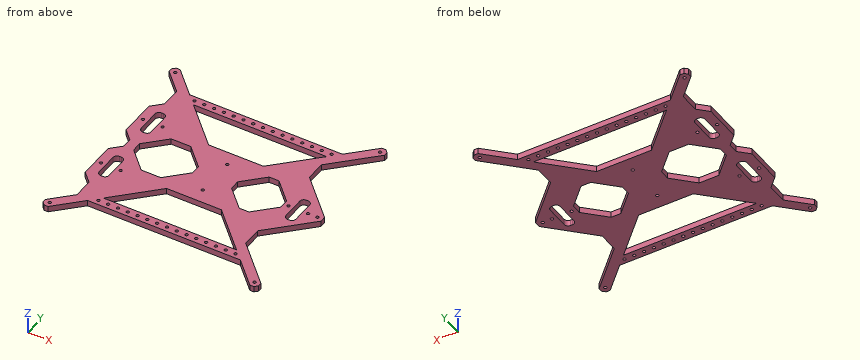
from build123d import *

# Parameters (mm, degrees)
MODEL_R                 = 1.5
SALIENTE_EXTRUIR1_DEPTH = 6
CROQUIS2_R              = 1.5
CROQUIS2_R_2            = 0.241728607
CORTAR_EXTRUIR1_DEPTH   = 7


with BuildPart() as part:
    # Model → Saliente-Extruir1 (new body)
    with BuildSketch(Plane.XY):
        Polygon((-105, 110), (-107, 110), (-110, 107), (-110, 105), (-110, 103), (-90, 83), (-90, 63), (-100, 53), (-100, 15), (-90, 5), (-90, -5), (-100, -15), (-100, -53), (-90, -63), (-90, -83), (-110, -103), (-110, -107), (-107, -110), (-105, -110), (-103, -110), (-78, -85), (78, -85), (103, -110), (105, -110), (107, -110), (110, -107), (110, -103), (90, -83), (70, -63), (70, -43), (90, -23), (110, -3), (110, 3), (90, 23), (70, 43), (70, 63), (110, 103), (110, 106), (110, 107), (107, 110), (103, 110), (80, 87), (78, 85), (-78, 85), (-103, 110), align=None)
        with Locations((104.5, 0)):
            Circle(MODEL_R, mode=Mode.SUBTRACT)
        with Locations((-95, 35)):
            Circle(MODEL_R, mode=Mode.SUBTRACT)
        with Locations((-75, 35)):
            Circle(MODEL_R, mode=Mode.SUBTRACT)
        with Locations((-95, -35)):
            Circle(MODEL_R, mode=Mode.SUBTRACT)
        with Locations((-75, -35)):
            Circle(MODEL_R, mode=Mode.SUBTRACT)
        with Locations((95, 0)):
            Circle(MODEL_R, mode=Mode.SUBTRACT)
        with Locations((75, 0)):
            Circle(MODEL_R, mode=Mode.SUBTRACT)
        with Locations((-104.5, 104.5)):
            Circle(MODEL_R, mode=Mode.SUBTRACT)
        with Locations((104.5, -104.5)):
            Circle(MODEL_R, mode=Mode.SUBTRACT)
        with Locations((104.5, 104.5)):
            Circle(MODEL_R, mode=Mode.SUBTRACT)
        with Locations((-104.5, -104.5)):
            Circle(MODEL_R, mode=Mode.SUBTRACT)
        with Locations((0, -20.5)):
            Circle(MODEL_R, mode=Mode.SUBTRACT)
        with Locations((0, 20.5)):
            Circle(MODEL_R, mode=Mode.SUBTRACT)
        Polygon((40, 47), (38, 45), (28, 35), (-28, 35), (-68, 75), (68, 75), align=None, mode=Mode.SUBTRACT)
        Polygon((28, -35), (-28, -35), (-68, -75), (68, -75), align=None, mode=Mode.SUBTRACT)
        Polygon((-80, 5), (-60, 25), (-40, 25), (-20, 5), (-20, -5), (-40, -25), (-60, -25), (-80, -5), align=None, mode=Mode.SUBTRACT)
        Polygon((50, 25), (70, 5), (70, -5), (50, -25), (40, -25), (20, -5), (20, 5), (40, 25), align=None, mode=Mode.SUBTRACT)
        with BuildLine():
            Line((-90, -46), (-90, -23))
            ThreePointArc((-90, -23), (-88.828427125, -20.171572875), (-86, -19))
            Line((-86, -19), (-84, -19))
            ThreePointArc((-84, -19), (-81.171572875, -20.171572875), (-80, -23))
            Line((-80, -23), (-80, -46))
            ThreePointArc((-80, -46), (-81.171572875, -48.828427125), (-84, -50))
            Line((-84, -50), (-86, -50))
            ThreePointArc((-86, -50), (-88.828427125, -48.828427125), (-90, -46))
        make_face(mode=Mode.SUBTRACT)
        with BuildLine():
            Line((-90, 24.007036896), (-90, 47.007036896))
            ThreePointArc((-90, 47.007036896), (-88.828427125, 49.835464021), (-86, 51.007036896))
            Line((-86, 51.007036896), (-84, 51.007036896))
            ThreePointArc((-84, 51.007036896), (-81.171572875, 49.835464021), (-80, 47.007036896))
            Line((-80, 47.007036896), (-80, 24.007036896))
            ThreePointArc((-80, 24.007036896), (-81.171572875, 21.178609771), (-84, 20.007036896))
            Line((-84, 20.007036896), (-86, 20.007036896))
            ThreePointArc((-86, 20.007036896), (-88.828427125, 21.178609771), (-90, 24.007036896))
        make_face(mode=Mode.SUBTRACT)
        with BuildLine():
            Line((80, -12.137123607), (80, 10.862876393))
            ThreePointArc((80, 10.862876393), (81.171572875, 13.691303518), (84, 14.862876393))
            Line((84, 14.862876393), (86, 14.862876393))
            ThreePointArc((86, 14.862876393), (88.828427125, 13.691303518), (90, 10.862876393))
            Line((90, 10.862876393), (90, -12.137123607))
            ThreePointArc((90, -12.137123607), (88.828427125, -14.965550732), (86, -16.137123607))
            Line((86, -16.137123607), (84, -16.137123607))
            ThreePointArc((84, -16.137123607), (81.171572875, -14.965550732), (80, -12.137123607))
        make_face(mode=Mode.SUBTRACT)
    extrude(amount=SALIENTE_EXTRUIR1_DEPTH)

    # Croquis2 → Cortar-Extruir1 (cut, through all)
    with BuildSketch(Plane(origin=(0, 0, 0), x_dir=(-1, 0, 0), z_dir=(0, 0, -1))):
        with Locations((-70, 80)):
            Circle(CROQUIS2_R)
        with Locations((-70, -80)):
            Circle(CROQUIS2_R)
        with Locations((-61.506705716, -90.733837273)):
            Circle(CROQUIS2_R_2)
        with Locations((-60, -80)):
            Circle(CROQUIS2_R)
        with Locations((-60, 80)):
            Circle(CROQUIS2_R)
        with Locations((-50, -80)):
            Circle(CROQUIS2_R)
        with Locations((-50, 80)):
            Circle(CROQUIS2_R)
        with Locations((-40, -80)):
            Circle(CROQUIS2_R)
        with Locations((-40, 80)):
            Circle(CROQUIS2_R)
        with Locations((-30, -80)):
            Circle(CROQUIS2_R)
        with Locations((-30, 80)):
            Circle(CROQUIS2_R)
        with Locations((-20, -80)):
            Circle(CROQUIS2_R)
        with Locations((-20, 80)):
            Circle(CROQUIS2_R)
        with Locations((-10, -80)):
            Circle(CROQUIS2_R)
        with Locations((-10, 80)):
            Circle(CROQUIS2_R)
        with Locations((0, -80)):
            Circle(CROQUIS2_R)
        with Locations((0, 80)):
            Circle(CROQUIS2_R)
        with Locations((10, -80)):
            Circle(CROQUIS2_R)
        with Locations((10, 80)):
            Circle(CROQUIS2_R)
        with Locations((20, -80)):
            Circle(CROQUIS2_R)
        with Locations((20, 80)):
            Circle(CROQUIS2_R)
        with Locations((30, -80)):
            Circle(CROQUIS2_R)
        with Locations((30, 80)):
            Circle(CROQUIS2_R)
        with Locations((40, -80)):
            Circle(CROQUIS2_R)
        with Locations((40, 80)):
            Circle(CROQUIS2_R)
        with Locations((50, -80)):
            Circle(CROQUIS2_R)
        with Locations((50, 80)):
            Circle(CROQUIS2_R)
        with Locations((60, -80)):
            Circle(CROQUIS2_R)
        with Locations((60, 80)):
            Circle(CROQUIS2_R)
        with Locations((70, -80)):
            Circle(CROQUIS2_R)
        with Locations((70, 80)):
            Circle(CROQUIS2_R)
    extrude(amount=-CORTAR_EXTRUIR1_DEPTH, mode=Mode.SUBTRACT)


solid = part.part
Geometry: final body of the model. Coordinates: model frame, mm. Coordinates: 2 decimals unless noted, no trailing zeros. Order: outer loops, then holes, each group sorted by start corner. A loop starts at its lowest first (then second) coordinate and runs counter-clockwise, first axis right, second up.
(1) First-contact query: pin 1 (2.5 mm diameter, centred on x = 70, y = -80, fed in from +Z); pin 2 (2 mm diameter, centred on x = 74, z = 2.5, fed in from +Y); pin 3 (3 mm diameter, centred on x = -32.5, z = 1.5, fed in from -Y); pin 4 (3 mm diameter, centred on x = 77.5, z = 1, fed in from +Y). Flat tips, straight axial feed; report the tip coordinate or a pass-through.
(2) Section query A-A (y = 90.5). Return the cut outline in (x, z), plus the area to 3 significant figures.
(3) Material intervals for probe 1 along Y at (x, z) = (-10, 4.3); probe 2 along Y at (x, z) = (-17, 4.6); probe 3 along Y at (x, z) = (56, 0.35), sorted ascending.
(4) Section query B-B (z = 3.4). State how many separate pieces and enclosed holes the cut face has, plus the area to 3 significant figures.
Solution:
1. pin 1: passes through
1. pin 2: stops at y = 85
1. pin 3: stops at y = -85
1. pin 4: stops at y = 86
2. outline: (-97.5, 0) - (-83.5, 0) - (-83.5, 6) - (-97.5, 6) - close; (83.5, 0) - (97.5, 0) - (97.5, 6) - (83.5, 6) - close
2. area: 168 mm2
3. probe 1: y = -85 to -81.5, -78.5 to -75, -35 to 35, 75 to 78.5, 81.5 to 85
3. probe 2: y = -85 to -75, -35 to 35, 75 to 85
3. probe 3: y = -85 to -75, -63 to -19, 19 to 63, 75 to 85
4. separate pieces: 1
4. enclosed holes: 50
4. area: 19,000 mm2
